Geometry check sheet. Reference: drawing and pictorial views, mm from the part's lowest x, y, z. Give positions to 0.01 mm unless a question says otherwise; leave off trailing zeros. Order: outer loops, then holes, each group sorted by start corner. A loop starts at its lowest first (then second) coordinate and runs counter-clockwise, first axis right, second up. Notation, with made-up numbers: M 7,-36.75 L 63,-36.75 A37 ccw 63,2.25 Z; hole C 63,32.5 d7. An arc over 180 degrees is marked long. Answer as CSV lines item,"result".
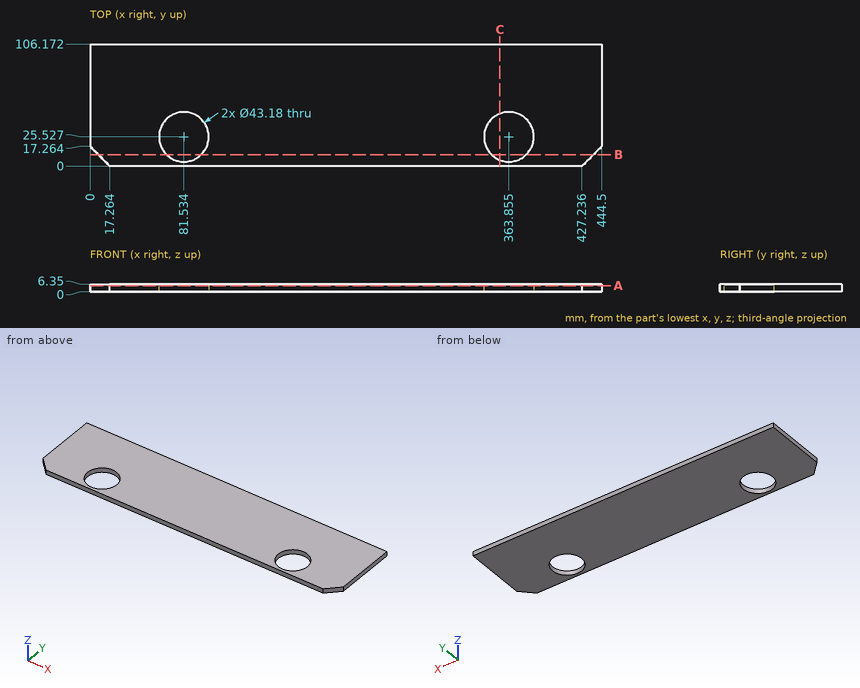
(1) Material ranges on line 1 (X direction, y = 38, z = 1.5) (1 decimal); line 2 (X direction, y = 26, z = 1.5); line 3 (Y direction, x = 370.5, z = 3.75) (1 decimal), recorded low to high.
The answers:
line 1,"x = 0 to 63.9, 99.2 to 346.2, 381.5 to 444.5"
line 2,"x = 0 to 59.95, 103.12 to 342.27, 385.44 to 444.5"
line 3,"y = 0 to 5, 46.1 to 106.2"
(2) Section check C-C on x = 356. Enter the section's corners in (y, z), then the cut area to 3 significant figures.
The answers:
outline,"M 0,0 L 5.42,0 L 5.42,6.35 L 0,6.35 Z; M 45.64,0 L 106.17,0 L 106.17,6.35 L 45.64,6.35 Z"
area,"419 mm2"
(3) Section check B-B on y = 10. State how many separate pieces and enclosed holes the cut face has, then the cut area to 3 significant figures.
The answers:
separate pieces,"3"
enclosed holes,"0"
area,"2,350 mm2"
(4) Section check A-A on z = 5.25. Enter the section's corners in (x, y) (1 decimal).
The answers:
outline,"M 0,17.3 L 17.3,0 L 427.2,0 L 444.5,17.3 L 444.5,106.2 L 0,106.2 Z; hole C 81.5,25.5 d43.2; hole C 363.9,25.5 d43.2"
